Work out the finished part from the listing and answer in its coordinate system (mm). A direction names the side the tool comes from. Give positions to 0.01 mm unless a question says otherwise; leave off trailing zeros. Write item = value, one per line. Start each with the question number.
1. Consider L1, parallel to X at y = 4.5, z = -2 (3 decimals); L2, parallel to X at y = 15.75, z = -2.5; L3, parallel to Z at x = 0.75, y = 2.5. Determine where each line is inside the solid, lowest interval first. Write a range as [from, to].
2. Flat-ended cylindrical pins translate along their axes: pin 1 Ø6 at (x, z) = (2.5, 0.5) entering from +Y; pin 2 Ø0.8 at (x, y) = (4.5, 17) entering from +Z (3 decimals); pin 3 Ø1.2 at (y, z) = (14, 1) entering from -X. Find the tip coordinate at first contact, or state that the pin passes through.
3. The mould has two halves that part along Z. Classify faces 6 (the face through (2.5, 15, -7)), 7 (the face through (-1.25, 15, -3)): released by +Z, released by -Z, zero draft, split by the parting line, or undercut.
4. Section A-A on y = 18 is taken. Give the number of separate pieces and of enclosed holes in the cut face, plus the area to 3 significant figures.
5. For faces 1 (the face through (0, 15, -0.875)), 2 (the face through (-4, 15, 0.375)), 3 (the face through (0, 5, 0.25)), 4 (the face through (3, 8, -6)), 5 (the face through (-1.75, 15, 2)), determine the directions among +Z, -Z, +X, -X, +Y, -Y from which every point of the face is accessible in a straight line to the end or side of a thin tool.
```python
from build123d import *

# Parameters (mm, degrees)
SKIZZE1_W                       = 10
SKIZZE1_H                       = 11
AUFSATZ_LINEAR_AUSTRAGEN1_DEPTH = 7
SKIZZE2_W                       = 1.5
SKIZZE2_H                       = 1
AUFSATZ_LINEAR_AUSTRAGEN2_DEPTH = 7
AUFSATZ_LINEAR_AUSTRAGEN3_DEPTH = 4
SKIZZE4_W                       = 5
SKIZZE4_H                       = 1.5
SCHNITT_LINEAR_AUSTRAGEN1_DEPTH = 12
AUFSATZ_LINEAR_AUSTRAGEN4_DEPTH = 2.5
SKIZZE6_W                       = 3.75
SKIZZE6_H                       = 3.75
SCHNITT_LINEAR_AUSTRAGEN2_DEPTH = 10
LINEARES_MUSTER1_COUNT          = 3
LINEARES_MUSTER1_PITCH          = 4.25
LINEARES_MUSTER1_COUNT_DIR2     = 2
LINEARES_MUSTER1_PITCH_DIR2     = 4.25
SKIZZE7_W                       = 3.5
SKIZZE7_H                       = 3.5
AUFSATZ_LINEAR_AUSTRAGEN5_DEPTH = 9
LINEARES_MUSTER2_COUNT          = 3
LINEARES_MUSTER2_PITCH          = 4.25
LINEARES_MUSTER2_COUNT_DIR2     = 2
LINEARES_MUSTER2_PITCH_DIR2     = 4.25
AUFSATZ_LINEAR_AUSTRAGEN7_DEPTH = 9
LINEARES_MUSTER4_COUNT          = 3
LINEARES_MUSTER4_PITCH          = 4.25
LINEARES_MUSTER4_COUNT_DIR2     = 2
LINEARES_MUSTER4_PITCH_DIR2     = 4.25
SCHNITT_LINEAR_AUSTRAGEN4_DEPTH = 21
LINEARES_MUSTER6_COUNT          = 3
LINEARES_MUSTER6_PITCH          = 4.25
LINEARES_MUSTER6_COUNT_DIR2     = 2
LINEARES_MUSTER6_PITCH_DIR2     = 4.25


with BuildPart() as part:
    # Skizze1 → Aufsatz-Linear austragen1 (new body, symmetric)
    with BuildSketch(Plane(origin=(0, 0, 0), x_dir=(0, 0, -1), z_dir=(1, 0, 0))):
        with Locations((0, 5.5)):
            Rectangle(SKIZZE1_W, SKIZZE1_H)
    extrude(amount=AUFSATZ_LINEAR_AUSTRAGEN1_DEPTH, both=True)

    # Skizze2 → Aufsatz-Linear austragen2 (add, symmetric)
    with BuildSketch(Plane(origin=(0, 0, 0), x_dir=(0, 0, -1), z_dir=(1, 0, 0))):
        with Locations((-5.75, 0.5)):
            Rectangle(SKIZZE2_W, SKIZZE2_H)
        with Locations((5.75, 0.5)):
            Rectangle(SKIZZE2_W, SKIZZE2_H)
    extrude(amount=AUFSATZ_LINEAR_AUSTRAGEN2_DEPTH, both=True)

    # Skizze3 → Aufsatz-Linear austragen3 (add, symmetric)
    with BuildSketch(Plane(origin=(0, 0, 0), x_dir=(0, 0, -1), z_dir=(1, 0, 0))):
        with BuildLine():
            Line((5, 11), (5.571713615, 11))
            ThreePointArc((5.571713615, 11), (5.836038655, 10.149642784), (6.535856807, 9.598979842))
            ThreePointArc((6.535856807, 9.598979842), (7.23567496, 9.048316901), (7.5, 8.197959685))
            Line((7.5, 8.197959685), (7.5, 5.197959685))
            Line((7.5, 5.197959685), (8.5, 4))
            Line((8.5, 4), (8.5, 2))
            Line((8.5, 2), (6.5, 2))
            Line((6.5, 2), (6.5, 8))
            Line((6.5, 8), (5, 8))
            Line((5, 8), (5, 11))
        make_face()
    extrude(amount=AUFSATZ_LINEAR_AUSTRAGEN3_DEPTH, both=True)

    # Skizze4 → Schnitt-Linear austragen1 (cut, through all)
    with BuildSketch(Plane.XZ):
        with Locations((0, -5.75)):
            Rectangle(SKIZZE4_W, SKIZZE4_H)
    extrude(amount=-SCHNITT_LINEAR_AUSTRAGEN1_DEPTH, mode=Mode.SUBTRACT)

    # Skizze5 → Aufsatz-Linear austragen4 (add, symmetric)
    with BuildSketch(Plane(origin=(0, 0, 0), x_dir=(0, 0, -1), z_dir=(1, 0, 0))):
        Polygon((8.123516438, 4.451012129), (8.123516438, 19.870653012), (7.136310593, 21), (6.136310593, 21), (4.623516438, 19.677608169), (4.623516438, 17.677608169), (6.123516438, 17.677608169), (6.5, 8), (6.5, 2), align=None)
    extrude(amount=AUFSATZ_LINEAR_AUSTRAGEN4_DEPTH, both=True)

    # Skizze6 → Schnitt-Linear austragen2 (cut)
    with BuildSketch(Plane.XZ):
        with Locations((-4.25, -2.125)):
            Rectangle(SKIZZE6_W, SKIZZE6_H)
    schnitt_linear_austragen2 = extrude(amount=-SCHNITT_LINEAR_AUSTRAGEN2_DEPTH, mode=Mode.SUBTRACT)

    # Lineares Muster1: Schnitt-Linear austragen2 3 × 2
    with Locations(*[(i * LINEARES_MUSTER1_PITCH, 0, j * LINEARES_MUSTER1_PITCH_DIR2) for i in range(LINEARES_MUSTER1_COUNT) for j in range(LINEARES_MUSTER1_COUNT_DIR2) if (i, j) != (0, 0)]):
        add(schnitt_linear_austragen2, mode=Mode.SUBTRACT)

    # Skizze7 → Aufsatz-Linear austragen5 (add)
    with BuildSketch(Plane(origin=(0, 11, 0), x_dir=(1, 0, 0), z_dir=(0, 1, 0))):
        with Locations((-4.25, -2.125)):
            Rectangle(SKIZZE7_W, SKIZZE7_H)
    aufsatz_linear_austragen5 = extrude(amount=AUFSATZ_LINEAR_AUSTRAGEN5_DEPTH)

    # Lineares Muster2: Aufsatz-Linear austragen5 3 × 2, 4 skipped
    with Locations(*[(i * LINEARES_MUSTER2_PITCH, 0, -j * LINEARES_MUSTER2_PITCH_DIR2) for i in range(LINEARES_MUSTER2_COUNT) for j in range(LINEARES_MUSTER2_COUNT_DIR2) if (i, j) not in ((0, 0), (0, 1), (1, 0), (1, 1), (2, 0))]):
        add(aufsatz_linear_austragen5)

    # Skizze10 → Aufsatz-Linear austragen7 (add)
    with BuildSketch(Plane(origin=(0, 11, 0), x_dir=(1, 0, 0), z_dir=(0, 1, 0))):
        Polygon((-2.5, 1.375), (-3.5, 0.375), (-5, 0.375), (-6, 1.375), (-6, 3.875), (-2.5, 3.875), align=None)
    aufsatz_linear_austragen7 = extrude(amount=AUFSATZ_LINEAR_AUSTRAGEN7_DEPTH)

    # Lineares Muster4: Aufsatz-Linear austragen7 3 × 2, 2 skipped
    with Locations(*[(i * LINEARES_MUSTER4_PITCH, 0, j * LINEARES_MUSTER4_PITCH_DIR2) for i in range(LINEARES_MUSTER4_COUNT) for j in range(LINEARES_MUSTER4_COUNT_DIR2) if (i, j) not in ((0, 0), (0, 1), (2, 0))]):
        add(aufsatz_linear_austragen7)

    # Skizze12 → Schnitt-Linear austragen4 (cut, through all)
    with BuildSketch(Plane(origin=(0, 20, 0), x_dir=(1, 0, 0), z_dir=(0, 1, 0))):
        Polygon((-3.75, 0.875), (-3, 1.625), (-3, 3.375), (-5.5, 3.375), (-5.5, 1.625), (-4.75, 0.875), align=None)
    schnitt_linear_austragen4 = extrude(amount=-SCHNITT_LINEAR_AUSTRAGEN4_DEPTH, mode=Mode.SUBTRACT)

    # Lineares Muster6: Schnitt-Linear austragen4 3 × 2
    with Locations(*[(i * LINEARES_MUSTER6_PITCH, 0, j * LINEARES_MUSTER6_PITCH_DIR2) for i in range(LINEARES_MUSTER6_COUNT) for j in range(LINEARES_MUSTER6_COUNT_DIR2) if (i, j) != (0, 0)]):
        add(schnitt_linear_austragen4, mode=Mode.SUBTRACT)


solid = part.part
```
Verdict:
q1.L1 = [-7, -6.125], [-2.375, -1.875], [1.875, 2.375], [6.125, 7]
q1.L2 = [-6, -5.5], [-3, -2.5], [-1.75, -1.25], [1.25, 1.75], [2.5, 3], [5.5, 6]
q1.L3 = [-8.5, -6.5], [-5, -4], [-0.25, 0.25], [4, 5]
q2.pin_1 = 20
q2.pin_2 = 3.875
q2.pin_3 = -6
q3.face_6 = zero draft
q3.face_7 = undercut
q4.separate_pieces = 7
q4.enclosed_holes = 6
q4.area = 52.9 mm2
q5.face_1 = +Y, -Y
q5.face_2 = +X, -X, +Y
q5.face_3 = -Y
q5.face_4 = +X, -X
q5.face_5 = +Z, +Y
